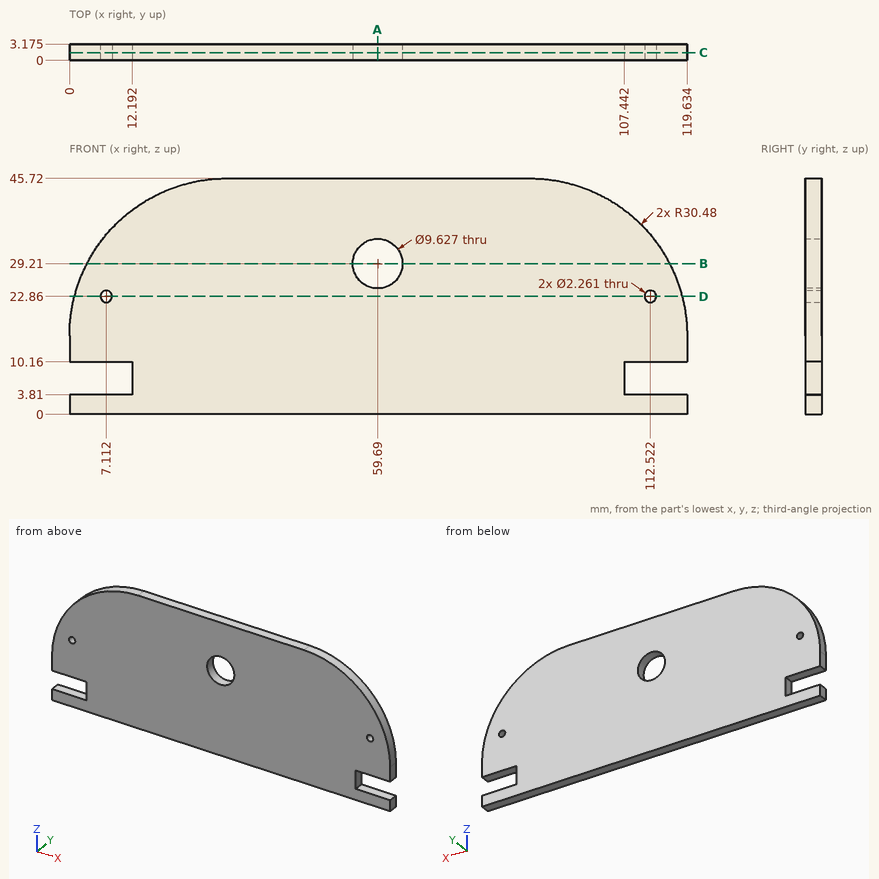
Design review of the part shown in the three views and the two pictorial views. Dimensions are in mm from the part's minimum x, y and z. Give positions to 0.01 mm unless a question says otherwise; leave off trailing zeros. Loops run counter-clockwise (first coordinate to the right, second up) from the corner with the lowest first, then second, coordinate; pieces in that order, holes last. Notation, with made-up numbers: (32.5, 52.25) - (80.5, 52.25) arc R15 cw to (80.5, 74.25) - close; hole circle Ø1 at (79, 77). An arc over 180 degrees is marked (long way). Write item = value, one per line.
1) Clearance check with flat-ended pins moving along their axes: pin 1 Ø11 at (x, z) = (59.69, 29.21) entering from +Y (3 decimals); pin 2 Ø1 at (y, z) = (2, 8) entering from +X; pin 3 Ø1.6 at (y, z) = (1.5, 8.5) entering from -X; pin 4 Ø1.6 at (x, y) = (112.5, 2) entering from +Z. State where each tip first meets the part, or that it passes through.
Result sheet:
pin_1 = 3.175
pin_2 = 107.44
pin_3 = 12.19
pin_4 = 35.75
2) Take a section at C-C on y = 1.5. State the section outline as (x, z) points.
Result sheet:
outline = (0, 0) - (119.63, 0) - (119.63, 3.81) - (107.44, 3.81) - (107.44, 10.16) - (119.63, 10.16) - (119.63, 15.24) arc R30.48 ccw to (89.15, 45.72) - (30.48, 45.72) arc R30.48 ccw to (0, 15.24) - (0, 10.16) - (12.19, 10.16) - (12.19, 3.81) - (0, 3.81) - close; hole circle Ø2.26 at (7.11, 22.86); hole circle Ø9.63 at (59.69, 29.21); hole circle Ø2.26 at (112.52, 22.86)
3) Take a section at B-B on z = 29.21. State the section outline as (x, y) points (1 decimal), and give its area (3 significant figures).
Result sheet:
outline = (3.4, 0) - (54.9, 0) - (54.9, 3.2) - (3.4, 3.2) - close; (64.5, 0) - (116.2, 0) - (116.2, 3.2) - (64.5, 3.2) - close
area = 328 mm2
4) To check wall thickness, follow line 1 (X direction, y = 1.05, z = 22.86) (1 decimal); line 2 (X direction, y = 2, z = 29.21) (1 decimal); line 3 (X direction, y = 1.1, z = 27) (1 decimal). State the ranges of each line that lie inside material, in increasing order.
Result sheet:
line_1 = 1 to 6, 8.2 to 111.4, 113.7 to 118.7
line_2 = 3.4 to 54.9, 64.5 to 116.2
line_3 = 2.4 to 55.4, 64 to 117.3
5) Take a section at D-D on z = 22.86. State the section outline as (x, y) points (1 decimal).
Result sheet:
outline = (1, 0) - (6, 0) - (6, 3.2) - (1, 3.2) - close; (8.2, 0) - (111.4, 0) - (111.4, 3.2) - (8.2, 3.2) - close; (113.7, 0) - (118.7, 0) - (118.7, 3.2) - (113.7, 3.2) - close
6) Take a section at A-A on x = 59.69. State the section outline as (y, z) points (1 decimal).
Result sheet:
outline = (0, 0) - (3.2, 0) - (3.2, 24.4) - (0, 24.4) - close; (0, 34) - (3.2, 34) - (3.2, 45.7) - (0, 45.7) - close
